Part print with two shaded views. Sizes in mm from the minimum x, y, z corner. A direction names the side the tool comes from. Round coordinates to 2 decimals unless told otherwise and drop trailing zeros. Order: outer loops, then holes, each group sorted by start corner. A loop starts at its lowest first (then second) coordinate and runs counter-clockwise, first axis right, second up. Notation, with made-up numbers: (64, 47.25) - (105, 47.25) arc R14 cw to (105, 58.25) - close; hole circle Ø8 at (4, -22.5). An arc over 180 degrees is marked (long way). Write item = value, one per line.
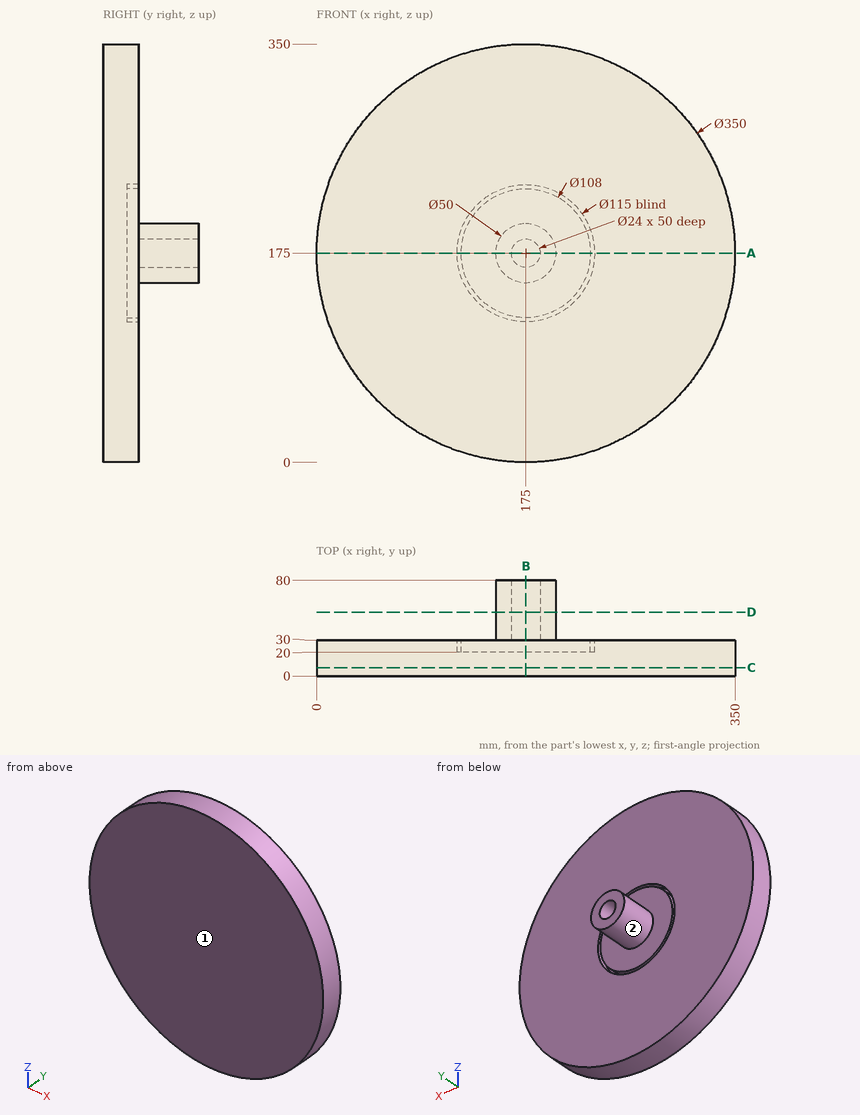
1) Wall check: line 1 along X through (y, z) = (23, 175); line 2 along X through (y, z) = (51.5, 175); line 3 along Y through (x, z) = (36.5, 83). Give the ranges that are in metal, low to high.
Conclusion:
line_1 = 0 to 117.5, 121 to 229, 232.5 to 350
line_2 = 150 to 163, 187 to 200
line_3 = 0 to 30
2) Flat gauge pins, fed straight in: pin 1 Ø1.5 at (x, z) = (263, 267) entering from +Y; pin 2 Ø1.5 at (x, y) = (196.5, 37.5) entering from -Z; pin 3 Ø3 at (y, z) = (10.5, 80) entering from +X. Where does each tip first touch, or does it go through?
Conclusion:
pin_1 = 30
pin_2 = 161.06
pin_3 = 322.93
3) Cut at B-B (x = 175). Write the cut outline in (y, z), and give its area (3 significant figures).
Conclusion:
outline = (0, 0) - (30, 0) - (30, 117.5) - (20, 117.5) - (20, 121) - (30, 121) - (30, 150) - (80, 150) - (80, 163) - (30, 163) - (30, 187) - (80, 187) - (80, 200) - (30, 200) - (30, 229) - (20, 229) - (20, 232.5) - (30, 232.5) - (30, 350) - (0, 350) - close
area = 11,700 mm^2
4) 3-axis set-ups, long thin cutter, end or side, ignore diameter. For the marked faces 1 and 2: which of +Z, -Z, +X, -X, +Y, -Y reach the whole face in a straight line?
Conclusion:
face_1 = +Z, -Z, +X, -X, -Y
face_2 = +Y
5) Cut at C-C (y = 7). Write the cut outline in (x, z), and give its area (3 significant figures).
Conclusion:
outline = circle Ø350 at (175, 175)
area = 96,200 mm^2
6) Cut at D-D (y = 53.5). Write the cut outline in (x, z).
Conclusion:
outline = circle Ø50 at (175, 175); hole circle Ø24 at (175, 175)
7) Cut at A-A (z = 175). Write the cut outline in (x, y).
Conclusion:
outline = (0, 0) - (350, 0) - (350, 30) - (232.5, 30) - (232.5, 20) - (229, 20) - (229, 30) - (200, 30) - (200, 80) - (187, 80) - (187, 30) - (163, 30) - (163, 80) - (150, 80) - (150, 30) - (121, 30) - (121, 20) - (117.5, 20) - (117.5, 30) - (0, 30) - close
